Geometry check sheet. Reference: the model listing, model coordinates, mm. Face numbers are marked on the shaded views. A direction names the side the tool comes from. Give positions to 0.01 mm unless a question says otherwise; leave off trailing zeros. Write each loop counter-clockwise with the first axis right and the second up, starting at its lowest first coordinate (ties: lowest second). Pieces come first, ordered by that corner, then holes. Notation, with made-up numbers: (13, 42) - (48, 42) arc R21 ccw to (48, 56) - close; hole circle Ø7 at (-33.75, 62). An arc over 180 degrees is marked (long way). Use a Markdown table: item, result.
```python
from build123d import *


with BuildPart() as f1:
    # F0 (on Top) → F1 (revolve)
    with BuildSketch(Plane.XY):
        Polygon((11.176, -1.27), (1.778, -1.27), (1.778, 0), (1.778, 0.35672), (0, 0.35672), (0, -0.91328), (-9.906, -1.397), (-9.906, -1.143), (-11.176, -1.143), (-11.176, -1.778), (-4.826, -1.778), (-4.826, -2.54), (0, -2.54), (0, -4.953), (1.524, -4.953), (1.524, -2.54), (9.906, -2.54), (9.906, -1.778), (11.176, -1.778), align=None)
    revolve(axis=Axis((0.762, -4.953, 0), (-1, 0, 0)))


solid = f1.part
```
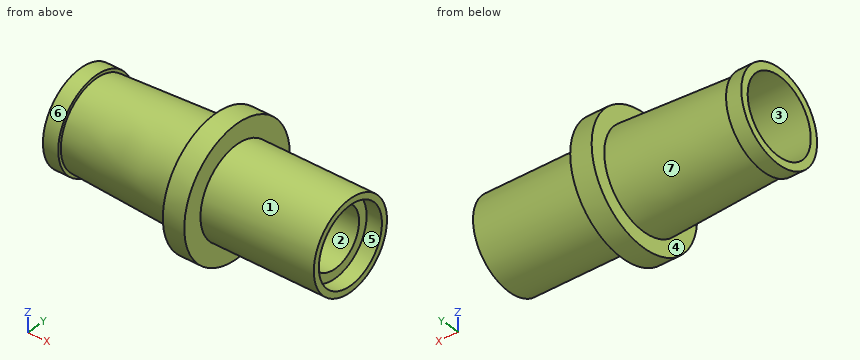
1) Set-up check for the marked faces 5, 6 and 7: record each of +Z, -Z, +X, -X, +Y, -Y from which the full face is reachable in a straight line by a thin tool's end or side.
Working result:
| item | result |
|---|---|
| face 5 | +X |
| face 6 | -X |
| face 7 | none |
2) Section check D-D on x = -9. Record the boundary of the cut face in (y, z) (3 decimals), then the cut area to 3 significant figures.
Working result:
| item | result |
|---|---|
| outline | circle Ø7.2 at (-4.953, 0); hole circle Ø6.35 at (-4.953, 0) |
| area | 9.05 mm² |
3) Section check A-A on x = 9.25. Record the boundary of the cut face in (y, z).
Working result:
| item | result |
|---|---|
| outline | circle Ø7.37 at (-4.95, 0); hole circle Ø4.83 at (-4.95, 0) |
4) Depth check by flat-ended pin: P1, Ø4, axis at y = -4.5, z = -1, coming from the -X side; P2, Ø2, axis at y = -1, z = 0, coming from the +X side; P3, Ø2, axis at y = -1, z = 3, coming from the +X side; P4, Ø2.5, axis at y = -5.5, z = 0.5, coming from the +X side. Enter the tip coordinate at first touch or a pass-through.
Working result:
| item | result |
|---|---|
| P1 | stops at x = -4.83 |
| P2 | stops at x = 11.18 |
| P3 | stops at x = 1.78 |
| P4 | stops at x = 1.52 |
5) Material ranges on L1, parallel to Y at x = 10.9, z = 0; L2, parallel to Z at x = 3, y = -6.5; L3, parallel to Y at x = -1.75, z = -1, recorded low to high. Write a range as from..to.
Working result:
| item | result |
|---|---|
| L1 | y = -8.64..-8.13, -1.78..-1.27 |
| L2 | z = -3.34..-1.85, 1.85..3.34 |
| L3 | y = -8.78..-7.15, -2.76..-1.13 |
6) Mould release check, pull along Y, two halves, no side actions. Record for the marked faces 1, 2, 3 and 4: pulls with the +Y half, pulls with the -Y half, needs draft (parallel to the pull), parting line crosses it, or undercut.
Working result:
| item | result |
|---|---|
| face 1 | parting line crosses it |
| face 2 | undercut |
| face 3 | undercut |
| face 4 | needs draft |
7) Section check C-C on x = 0.75. Record the boundary of the cut face in (y, z), then the cut area to 3 significant figures.
Working result:
| item | result |
|---|---|
| outline | circle Ø10.62 at (-4.95, 0) |
| area | 88.6 mm² |
